Source: CAD feature listing. Evaluate the final solid. Frame: model axes, mm. A direction names the side the tool comes from. Give positions to 0.01 mm unless a question says otherwise; leave off trailing zeros. Loops run counter-clockwise (first coordinate to the right, second up) from the corner with the lowest first, then second, coordinate; pieces in that order, holes last.
```python
from build123d import *

# Parameters (mm, degrees)
PARALLELEPIPEDOBLOCCO_DEPTH  = 20
SCHIZZO2_R                   = 11
SCHIZZO2_R_2                 = 6
FORITUBIMOTORI_DEPTH         = 46.656352242
SCHIZZO3_W                   = 7.05
SCHIZZO3_H                   = 15
SPAZIOMOVIMENTOLEVETTA_DEPTH = 46.656352242


with BuildPart() as part:
    # Schizzo1 → ParallelepipedoBlocco (new body)
    with BuildSketch(Plane.XY):
        Polygon((-30.55, -25), (30.55, -25), (32.55, -25), (32.55, 17), (-32.55, 17), (-32.55, -25), align=None)
    extrude(amount=PARALLELEPIPEDOBLOCCO_DEPTH)

    # Schizzo2 → ForiTubiMotori (cut, through all)
    with BuildSketch(Plane.XY.offset(20)):
        with Locations((-16.665, 0)):
            Circle(SCHIZZO2_R)
        with Locations((16.665, 0)):
            Circle(SCHIZZO2_R)
        with Locations((0, -15)):
            Circle(SCHIZZO2_R_2)
    extrude(amount=-FORITUBIMOTORI_DEPTH, mode=Mode.SUBTRACT)

    # Schizzo3 → SpazioMovimentoLevetta (cut, through all)
    with BuildSketch(Plane.XY.offset(20)):
        with Locations((-29.025, -17.5)):
            Rectangle(SCHIZZO3_W, SCHIZZO3_H)
    extrude(amount=-SPAZIOMOVIMENTOLEVETTA_DEPTH, mode=Mode.SUBTRACT)


solid = part.part
```
(1) Section D-D, the plane y = -15. Return the cut outline in (x, z), then the cut area to 3 significant figures.
A:
outline: (-25.5, 0) - (-6, 0) - (-6, 20) - (-25.5, 20) - close; (6, 0) - (32.55, 0) - (32.55, 20) - (6, 20) - close
area: 921 mm2
(2) First-contact query: pin 1 (4.5 mm diameter, centred on y = -16, z = 11, fed in from -X). Flat tip, straight axial feed; report the tip coordinate or a pass-through.
A:
pin 1: stops at x = -25.5
(3) Section B-B, the plane x = 0. Return the cut outline in (y, z), then the cut area to 3 significant figures.
A:
outline: (-25, 0) - (-21, 0) - (-21, 20) - (-25, 20) - close; (-9, 0) - (17, 0) - (17, 20) - (-9, 20) - close
area: 600 mm2
(4) Section C-C, the plane z = 3.5. Return the cut outline in (x, y) (3 decimals).
A:
outline: (-32.55, -10) - (-25.5, -10) - (-25.5, -25) - (32.55, -25) - (32.55, 17) - (-32.55, 17) - close; hole circle Ø22 at (-16.665, 0); hole circle Ø12 at (0, -15); hole circle Ø22 at (16.665, 0)
(5) Reachability of faces 1 (the flat face through (-25.5, -18, 10)), 2 (the flat face through (0, -4, 20)) from +Z, -Z, +X, -X, +Y, -Y: full face, straight path, thin tool, end or side. Return the list, or none.
A:
face 1: +Z, -Z, -X, -Y
face 2: +Z, +X, -X, +Y, -Y
(6) Mould query, pull axis Y, two halves, no side actions, for faces 3 (the flat face through (0, 17, 10)), 4 (the flat face through (0, -4, 0)), 5 (the cylindrical face through (-0.78, -9.05, 10.14)), 6 (the flat face through (-29, -10, 10)). Classes: pulls with the +Y half, pulls with the -Y half, needs draft (parallel to the pull), parting line crosses it, or undercut.
A:
face 3: pulls with the +Y half
face 4: needs draft
face 5: undercut
face 6: pulls with the -Y half
(7) Ray query, line 1 along X through (y, z) = (-5, 14.75); line 2 along X through (y, z) = (-1, 13.75); line 3 along Y through (x, z) = (0, 7). Return the intervals inside material, ascending.
A:
line 1: x = -32.55 to -26.46, -6.87 to 6.87, 26.46 to 32.55
line 2: x = -32.55 to -27.62, -5.71 to 5.71, 27.62 to 32.55
line 3: y = -25 to -21, -9 to 17
(8) Section A-A, the plane y = 0. Return the cut outline in (x, z) (3 decimals), then the cut area to 3 significant figures.
A:
outline: (-32.55, 0) - (-27.665, 0) - (-27.665, 20) - (-32.55, 20) - close; (-5.665, 0) - (5.665, 0) - (5.665, 20) - (-5.665, 20) - close; (27.665, 0) - (32.55, 0) - (32.55, 20) - (27.665, 20) - close
area: 422 mm2
